from build123d import *

# Parameters (mm, degrees)
SKETCH_1_W          = 160
SKETCH_1_H          = 120
EXTRUDE_1_DEPTH     = 10
SKETCH_2_W          = 85
SKETCH_2_H          = 74
CUT_EXTRUDE_1_DEPTH = 6
SKETCH_3_R          = 1.65
CUT_EXTRUDE_2_DEPTH = 101.498756211


with BuildPart() as part:
    # 草图1 → 凸台-拉伸1 (new body)
    with BuildSketch(Plane.XY):
        Rectangle(SKETCH_1_W, SKETCH_1_H)
    extrude(amount=EXTRUDE_1_DEPTH)

    # 草图2 → 切除-拉伸1 (cut)
    with BuildSketch(Plane.XY.offset(10)):
        Rectangle(SKETCH_2_W, SKETCH_2_H)
    extrude(amount=-CUT_EXTRUDE_1_DEPTH, mode=Mode.SUBTRACT)

    # 草图3 → 切除-拉伸2 (cut, through all)
    with BuildSketch(Plane(origin=(0, 0, 0), x_dir=(-1, 0, 0), z_dir=(0, 0, -1))):
        with Locations((-70, 40)):
            Circle(SKETCH_3_R)
        with Locations((-70, 20)):
            Circle(SKETCH_3_R)
        with Locations((-70, 0)):
            Circle(SKETCH_3_R)
        with Locations((-70, -20)):
            Circle(SKETCH_3_R)
        with Locations((-70, -40)):
            Circle(SKETCH_3_R)
    cut_extrude_2 = extrude(amount=-CUT_EXTRUDE_2_DEPTH, mode=Mode.SUBTRACT)

    # 镜向1: 切除-拉伸2 across plane
    add(cut_extrude_2.mirror(Plane(origin=(0, 0, 0), x_dir=(0, 0, 1), z_dir=(1, 0, 0))), mode=Mode.SUBTRACT)


solid = part.part
Model file for the job. Use its own axes, mm. A direction names the side the tool comes from. Coordinates: 2 decimals unless noted, no trailing zeros. Loops run counter-clockwise (first coordinate to the right, second up) from the corner with the lowest first, then second, coordinate; pieces in that order, holes last. Notation, with made-up numbers: (42, 82) -> (97, 82) arc R10 ccw to (97, 92) -> close; hole circle Ø3 at (16.25, 19). An arc over 180 degrees is marked (long way). Use one line per item in the form item = value. Start each with the question number.
(1) Tool access for faces 1 (the cylindrical face through (71.216, -18.885, 4.93)), 2 (the flat face through (42.5, -1, 7)): list every direction of +Z, -Z, +X, -X, +Y, -Y with a clear straight run to the whole face (end or side of a thin tool).
(2) Cut at B-B on z = 5.75. Give the number of separate pieces and of enclosed holes in the cut face, and give its area (3 significant figures).
(3) Cut at C-C on y = -40. Give the cut face in (x, z).
(4) Pull direction X, two halves, no side cores. Call faces 3 (the flat face through (-80, -1, 5)), 4 (the cylindrical face through (71.216, 21.115, 4.93)), 5 (the flat face through (-1, 41, 10)): pulls with the +X half, pulls with the -X half, needs draft (parallel to the pull), parting line crosses it, or undercut.
(5) Cut at A-A on x = -70. Give the cut face in (y, z).
(6) Flat gauge pins, fed straight in: pin 1 (5 mm diameter, centred on x = 8, y = -18, fed in from +Z); pin 2 (2.5 mm diameter, centred on x = 70, y = -20, fed in from -Z). Where does each tip first touch, or does it go through?
(7) Cut at D-D on x = -2. Give the cut face in (y, z).
(8) Probe probe 1 along Y at (x, z) = (70, 3); probe 2 along X at (y, z) = (-6, 5); probe 3 along X at (y, z) = (-21.5, 7). List the from-to ranges inside material, lowest first. Write a range as from..to.
Values:
q1.face_1 = +Z, -Z
q1.face_2 = +Z
q2.separate_pieces = 1
q2.enclosed_holes = 11
q2.area = 12,800 mm2
q3.outline = (-80, 0) -> (-71.65, 0) -> (-71.65, 10) -> (-80, 10) -> close; (-68.35, 0) -> (68.35, 0) -> (68.35, 10) -> (-68.35, 10) -> close; (71.65, 0) -> (80, 0) -> (80, 10) -> (71.65, 10) -> close
q4.face_3 = pulls with the -X half
q4.face_4 = undercut
q4.face_5 = needs draft
q5.outline = (-60, 0) -> (-41.65, 0) -> (-41.65, 10) -> (-60, 10) -> close; (-38.35, 0) -> (-21.65, 0) -> (-21.65, 10) -> (-38.35, 10) -> close; (-18.35, 0) -> (-1.65, 0) -> (-1.65, 10) -> (-18.35, 10) -> close; (1.65, 0) -> (18.35, 0) -> (18.35, 10) -> (1.65, 10) -> close; (21.65, 0) -> (38.35, 0) -> (38.35, 10) -> (21.65, 10) -> close; (41.65, 0) -> (60, 0) -> (60, 10) -> (41.65, 10) -> close
q6.pin_1 = 4
q6.pin_2 = through
q7.outline = (-60, 0) -> (60, 0) -> (60, 10) -> (37, 10) -> (37, 4) -> (-37, 4) -> (-37, 10) -> (-60, 10) -> close
q8.probe_1 = -60..-41.65, -38.35..-21.65, -18.35..-1.65, 1.65..18.35, 21.65..38.35, 41.65..60
q8.probe_2 = -80..-42.5, 42.5..80
q8.probe_3 = -80..-70.69, -69.31..-42.5, 42.5..69.31, 70.69..80
